Read the model definition and answer for the solid it produces. Units are mm, in the model's axes. Face numbers are marked on the shaded views. A direction names the side the tool comes from. Round coordinates to 2 decimals unless told otherwise and drop trailing zeros. Order: outer loops, then holes, each group sorted by start corner. A loop starts at its lowest first (then second) coordinate and runs counter-clockwise, first axis right, second up. Notation, with made-up numbers: M 48,46 L 88,46 A20 ccw 88,77 Z; hole C 81,-36.75 d5. An arc over 180 degrees is marked long. Answer as CSV lines item,"result".
Autodesk Inventor part; units mm, degrees
ref_plane "Work Plane4" through (-6.25, 2, 7) normal (0, 1, 0) x (1, 0, 0)
ref_plane "YZ Plane" through (0, 0, 0) normal (1, 0, 0) x (0, 1, 0)
ref_plane "XZ Plane" through (0, 0, 0) normal (0, 1, 0) x (-1, 0, 0)
sketch "Sketch14" plane through (0, 0, 0) normal (0, 0, 1) x (1, 0, 0)
  circle A0 centre (0, 0) radius 3.5
  line L0 (-1.25, -3.2692) -> (1.25, -3.2692)
  line L1 (1.25, -3.2692) -> (1.25, -18.2692)
  line L2 (1.25, -18.2692) -> (-1.25, -18.2692)
  line L3 (-1.25, -18.2692) -> (-1.25, -3.2692)
  arc A1 (-1.25, -6.4952) -> (-2.75, -2.1651) centre (-8.25, -6.4952) ccw
  arc A2 (2.75, -2.1651) -> (1.25, -6.4952) centre (8.25, -6.4952) ccw
  line L4 (-6.25, 5) -> (6.25, 5)
  line L5 (6.25, 5) -> (6.25, -18.2692)
  line L6 (6.25, -18.2692) -> (-6.25, -18.2692)
  line L7 (-6.25, -18.2692) -> (-6.25, 5)
  point P0 (-1.25, -18.2692)
  point P1 (1.25, -18.2692)
  point P2 (-1.25, -18.2692)
  dimension "d67" = 7
  dimension "d68" = 2.5
  dimension "d69" = 7
  dimension "d70" = 7
  dimension "d71" = 15
  dimension "d72" = 5
  dimension "d73" = 5
  dimension "d74" = 5
extrude "Extrusion8" add sketch "Sketch14" along normal blind 7 contours A0 A1 L3 L6 L7 L4 L5 L1 A2
extrude "Extrusion9" add sketch "Sketch14" against normal blind 8
hole "Hole12" at (0, 0, 0) direction (0, 0, -1) diameter 4 end through all
ref_plane "Work Plane4" through (-6.25, 2, 7) normal (0, 1, 0) x (1, 0, 0)
sketch "Sketch18" plane through (-6.25, 5, 7) normal (0, 1, 0) x (1, 0, 0)
  line L0 (12.5, 0) -> (12.5, 15)
  line L1 (12.5, 7) -> (20.5, 7)
  line L2 (20.5, 7) -> (20.5, 15)
  line L3 (20.5, 15) -> (12.5, 15)
  line L4 (12.5, 15) -> (12.5, 0)
  line L5 (0, 15) -> (12.5, 15)
  line L6 (20.5, 7) -> (12.5, 15) construction
  line L7 (19.25, 12.5877) -> (19.25, 9.4123)
  line L8 (19.25, 9.4123) -> (16.5, 7.8246)
  line L9 (16.5, 7.8246) -> (13.75, 9.4123)
  line L10 (13.75, 9.4123) -> (13.75, 12.5877)
  line L11 (13.75, 12.5877) -> (16.5, 14.1754)
  line L12 (16.5, 14.1754) -> (19.25, 12.5877)
  point P0 (6.25, 7)
  point P1 (16.5, 11)
  point P2 (16.5, 11)
  point P3 (12.5, 13)
  dimension "d112" = 8
  dimension "d113" = 5.5
  dimension "d139" = 8
extrude "Extrusion13" add sketch "Sketch18" against normal blind 6 contours L0 L3 L2 L1 | L7 L8 L9 L10 L11 L12
hole "Hole16" at (10.25, 5, -4) direction (0, -1, 0) diameter 4 end through all
sketch "Sketch19" plane through (6.25, -18.2692, 7) normal (1, 0, 0) x (0, 0, -1)
  line L0 (0, 0) -> (0, 11.774)
  line L1 (7, 0) -> (7, 11.774)
  line L2 (7, 11.774) -> (0, 11.774)
  line L3 (0, 0) -> (0, 11.774)
  line L4 (7, 0) -> (0, 0)
  line L5 (15, 17.2692) -> (7, 17.2692)
  line L6 (11, 8.6346) -> (11, 0) construction
  line L7 (7, 0) -> (15, 0) construction
  line L8 (15, 17.2692) -> (15, 0) construction
  line L9 (11, 8.6346) -> (11, 17.2692) construction
  point P0 (7, 18.2692)
hole "Hole15" at (6.25, -9.6346, -4) direction (-1, 0, 0) diameter 3.4 end through all counterbore diameter 6.5 counterbore depth 2
sketch "Sketch20" plane through (6.25, -18.2692, 7) normal (1, 0, 0) x (0, 0, -1)
  line L0 (15, 17.2692) -> (15, 0)
  circle A0 centre (11, 8.6346) radius 3.25
  circle A1 centre (11, 8.6346) radius 1.7
  circle A2 centre (11, 8.6346) radius 3.25
  line L1 (11, 5.3846) -> (11, 11.8846)
  line L2 (11, 11.8846) -> (15, 11.8846)
  line L3 (15, 11.8846) -> (15, 5.3846)
  line L4 (15, 5.3846) -> (11, 5.3846)
  point P0 (7, 18.2692)
extrude "Extrusion14" cut sketch "Sketch20" against normal up to surface (2 mm away) contours L0 L4 A0 L2 | A0 L1 A1 | A1 L1 picked at (13.692, 8.2674) picked at (11.6055, 9.0776)
fillet "Fillet3" radius 2 9 edges at (14.25, -1, -4) (-6.25, 5, -0.5) (-6.25, -18.2692, -0.5) (6.25, -18.2692, -0.5) (-1.25, -18.2692, 3.5) (1.25, -18.2692, 3.5) (6.25, -1, -4) (14.25, 5, -4) (6.25, 5, 3.5)
equation "\"d69\" = d67"
equation "\"d70\" = d67"
equation "\"d73\" = d72"
properties part number "z belt clip"
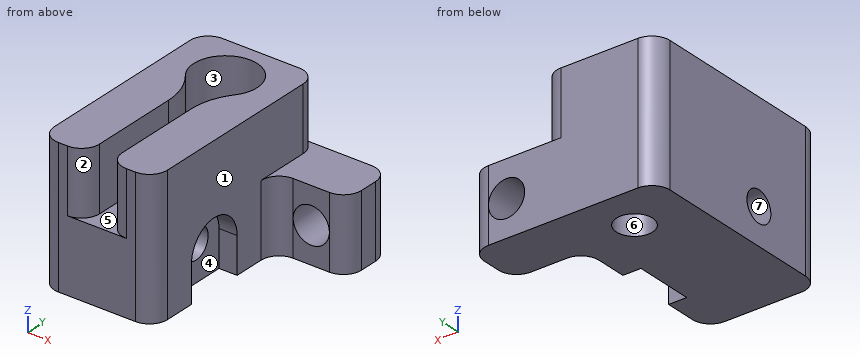
Item 1: A cutting plane is placed at C-C, the plane x = 0. Determine the outline of the cut face in (y, z), and give its area (3 significant figures).
Ans:
outline,"M -18.27,-8 L -2,-8 L -2,0 L -18.27,0 Z; M 2,-8 L 5,-8 L 5,7 L 3.5,7 L 3.5,0 L 2,0 Z; hole C -9.63,-4 d3.4"
area,"156 mm2"
Item 2: Determine the mould class of the marked faces 5, 6 and 7 for opening direction Z: +Z half, -Z half, draft (parallel to the pull), parting line (faces both ways), or undercut.
Ans:
face 5,"+Z half"
face 6,"draft"
face 7,"undercut"
Item 3: A cutting plane is placed at A-A, the plane x = 10.25. Determine the outline of the cut face in (y, z), and give its area (3 significant figures).
Ans:
outline,"M -1,-8 L 5,-8 L 5,-6 L -1,-6 Z; M -1,-2 L 5,-2 L 5,0 L -1,0 Z"
area,"24.0 mm2"
Item 4: A cutting plane is placed at D-D, the plane y = -10.25. Determine the outline of the cut face in (x, z).
Ans:
outline,"M -6.25,-8 L 4.25,-8 L 4.25,-5.58 L -6.25,-5.58 Z; M -6.25,-2.42 L 4.25,-2.42 L 4.25,-0.81 L 6.25,-0.81 L 6.25,7 L 1.25,7 L 1.25,0 L -1.25,0 L -1.25,7 L -6.25,7 Z"
Item 5: Flat-ended cylindrical pins translate along their axes: pin 1 (4 mm diameter, centred on x = 11, y = 3, fed in from +Z); pin 2 (1 mm diameter, centred on x = 5.5, z = -6, fed in from -Y); pin 3 (4.5 mm diameter, centred on y = -9.63, z = -4, fed in from +X). Find the tip coordinate at first contact, or state that the pin passes through.
Ans:
pin 1,"z = 0"
pin 2,"y = -18.12"
pin 3,"x = 4.25"
Item 6: A cutting plane is placed at B-B, the plane z = -2.75. Determine the outline of the cut face in (x, y).
Ans:
outline,"M -6.25,-16.27 A2 ccw -4.25,-18.27 L 4.25,-18.27 A2 ccw 6.25,-16.27 L 6.25,-12.63 L 4.25,-12.63 L 4.25,-10.79 L -6.25,-10.79 Z; M -6.25,-8.48 L 4.25,-8.48 L 4.25,-6.63 L 6.25,-6.63 L 6.25,-3 A2 cw 8.25,-1 L 8.69,-1 L 8.69,5 L -4.25,5 A2 ccw -6.25,3 Z; M 11.81,-1 L 12.25,-1 A2 ccw 14.25,1 L 14.25,3 A2 ccw 12.25,5 L 11.81,5 Z; hole C 0,0 d4"
Item 7: A tool of negligible diameter and unlimited length cuts with its end or side. For the marked faces 1, 2, 3 and 4, from which of +Z, -Z, +X, -X, +Y, -Y can it reach the whole face along a straight path? Write none if from no direction.
Ans:
face 1,"+Z, +X, -Y"
face 2,"+Z, -Y"
face 3,"+Z"
face 4,"-Z, +X"
Item 8: Find the intervals of material crossed by probe 1 along X at (y, z) = (0.3, -4); probe 2 along X at (y, z) = (0, 2.25); probe 3 along X at (y, z) = (-14.5, 0.75), in increasing order. Write a range as [from, to].
Ans:
probe 1,"[-6.25, -1.98], [1.98, 8.25], [12.25, 14.12]"
probe 2,"[-6.25, -3.5], [3.5, 6.25]"
probe 3,"[-6.25, -1.25], [1.25, 6.25]"
